Work out the finished part from the listing and answer in its coordinate system (mm). Coordinates: 2 decimals unless noted, no trailing zeros. Write each loop counter-clockwise with the first axis right and the second up, starting at its lowest first coordinate (ties: lowest second). Pieces come first, ordered by that corner, then holes. Notation, with made-up numbers: (19.25, 2) - (39.25, 2) arc R25 cw to (39.25, 34) - close; hole circle Ø4 at (77.25, 65.25). An arc over 180 degrees is marked (long way). Use a Markdown table: item, result. Add a question column.
(1) The part is cut by section A-A, the plane x = 0. Give the vertices of the cut face in (y, z).
(2) Find the intervals of material crossed by line 1 (Y direction, x = 0, z = -0.75); line 2 (Y direction, x = -3.5, z = -2.2); line 3 (X direction, y = 3.5, z = -1.5), in increasing order. Write a range as from..to.
(3) Given pin 1 Ø2 at (y, z) = (16, -3) entering from -X; pin 2 Ø1 at (x, z) = (-4.5, -2) entering from +Y; pin 3 Ø1.5 at (x, z) = (-13, -2) entering from -Y, each flat-ended and moving along its own axis, determine where each tip first touches the part or whether it passes through.
(4) The part is cut by section C-C, the plane z = -2.5. Give the vertices of the cut face in (x, y) (3 decimals), then the cut area to 3 significant figures.
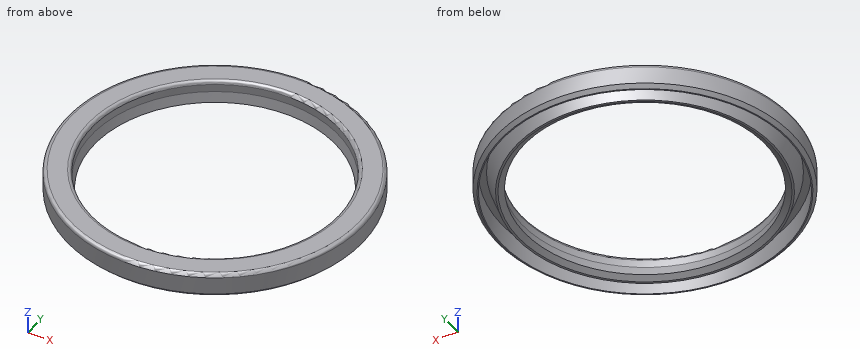
from build123d import *


with BuildPart() as part:
    # Sketch1 → Revolve1 (revolve)
    with BuildSketch(Plane(origin=(0, 0, 0), x_dir=(0, 0, -1), z_dir=(1, 0, 0)), mode=Mode.PRIVATE) as revolve1_sk:
        with BuildLine():
            Line((0, 18.05), (0, 20.56))
            ThreePointArc((0, 20.56), (0.146446609, 20.913553391), (0.5, 21.06))
            Line((0.5, 21.06), (3, 21.06))
            Line((3, 21.06), (3.5, 20.56))
            Line((3.5, 20.56), (3.5, 20.4))
            Line((3.5, 20.4), (0.5, 20.4))
            Line((0.5, 20.4), (0.5, 19.4))
            Line((0.5, 19.4), (3.5, 18.3))
            Line((3.5, 18.3), (3.5, 18))
            Line((3.5, 18), (3, 17.2))
            Line((3, 17.2), (1.6, 17.55))
            Line((1.6, 17.55), (0.5, 17.55))
            ThreePointArc((0.5, 17.55), (0.146446609, 17.696446609), (0, 18.05))
        make_face()
    revolve(revolve1_sk.sketch.rotate(Axis((0, 0, 0), (0, 0, -1)), 90), axis=Axis((0, 0, 0), (0, 0, -1)))


solid = part.part
Model answer:
| question | item | result |
|---|---|---|
| 1 | outline | (-21.06, -3) - (-20.56, -3.5) - (-20.4, -3.5) - (-20.4, -0.5) - (-19.4, -0.5) - (-18.3, -3.5) - (-18, -3.5) - (-17.2, -3) - (-17.55, -1.6) - (-17.55, -0.5) arc R0.5 ccw to (-18.05, 0) - (-20.56, 0) arc R0.5 ccw to (-21.06, -0.5) - close; (17.2, -3) - (18, -3.5) - (18.3, -3.5) - (19.4, -0.5) - (20.4, -0.5) - (20.4, -3.5) - (20.56, -3.5) - (21.06, -3) - (21.06, -0.5) arc R0.5 ccw to (20.56, 0) - (18.05, 0) arc R0.5 ccw to (17.55, -0.5) - (17.55, -1.6) - close |
| 2 | line 1 | -21.06..-20.4, -19.31..-17.55, 17.55..19.31, 20.4..21.06 |
| 2 | line 2 | -20.77..-20.1, -18.45..-17.04, 17.04..18.45, 20.1..20.77 |
| 2 | line 3 | -20.77..-20.1, -18.71..-17.2, 17.2..18.71, 20.1..20.77 |
| 3 | pin 1 | x = -14.78 |
| 3 | pin 2 | y = 20.68 |
| 3 | pin 3 | y = -17.13 |
| 4 | outline | circle Ø42.12 at (0, 0); circle Ø37.333 at (0, 0); hole circle Ø40.8 at (0, 0); hole circle Ø34.65 at (0, 0) |
| 4 | area | 238 mm^2 |
